Input: dimensioned drawing with shaded views. Units: mm. Origin: part minimum x, y, z. Round coordinates to 2 decimals unless told otherwise and drop trailing zeros. Loops run counter-clockwise (first coordinate to the right, second up) from the corner with the lowest first, then second, coordinate; pieces in that order, holes last. Notation, with made-up numbers: (74, 48) -> (87, 48) arc R17 cw to (87, 62) -> close; hole circle Ø2 at (-8, 81). An arc over 180 degrees is marked (long way). Answer as a JSON object with one key per item and string values.
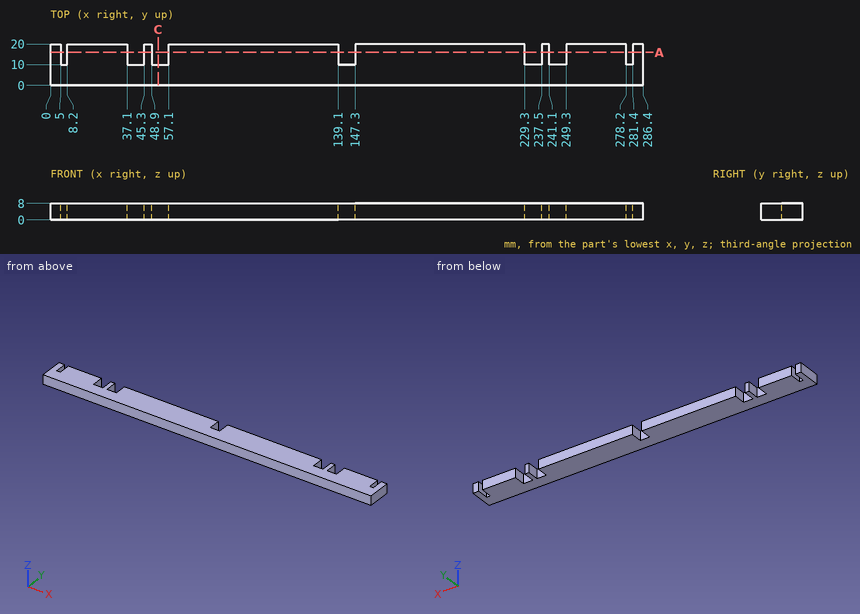
1) Ray query, probe 1 along Y at (x, z) = (236.5, 2.75). Return the intervals inside material, ascending.
Output:
{"probe 1": "y = 0 to 10"}
2) Section A-A, the plane y = 16. Count the separate pieces of the cut face and the enclosed holes in it, plus the area to 3 significant figures.
Output:
{"separate pieces": "8", "enclosed holes": "0", "area": "1,910 mm^2"}
3) Section C-C, the plane x = 52. Output: boundary loops of the cut face in (y, z), plus the area to 3 significant figures.
Output:
{"outline": "(0, 0) -> (10, 0) -> (10, 8) -> (0, 8) -> close", "area": "80.0 mm^2"}
4) Contact query for flat-ended pins moving along their axis: P1, Ø2.5, axis at y = 16.5, z = 4, coming from the -X side; P2, Ø1.6, axis at x = 279.5, z = 5.5, coming from the +Y side. Output: stop coordinate, or through.
Output:
{"P1": "stops at x = 0", "P2": "stops at y = 10"}
